The listing builds one solid part. Answer for the finished solid, in the listing's coordinates (mm). Give positions to 0.01 mm unless a question says otherwise; leave off trailing zeros. Order: outer loops, then holes, each group sorted by start corner. A loop starts at its lowest first (then second) coordinate and runs counter-clockwise, first axis right, second up. Notation, with made-up numbers: (20, -8.5) - (35, -8.5) arc R19 cw to (35, -0.5) - close; hole circle Ø6 at (-7.75, -5.75). An arc over 180 degrees is marked (long way). Write each question's results on one line, items separated by ' | '. Start each with the question number.
1. Determine the mould class of faces 1 (the face through (22.1, -9.1, 30)), 2 (the face through (-2.18, 16.61, 9.26)), 3 (the face through (0, 0, 1)) for opening direction Y: released by +Y, released by -Y, zero draft, split by the parting line, or undercut.
2. Section B-B (x = 0) is taken. Give the vertices of the cut face in (y, z), and give its area (3 significant figures).
3. Section C-C (z = 13) is taken. State how many separate pieces and enclosed holes the cut face has, and give its area (3 significant figures).
4. Flat-ended cylindrical pins translate along their axes: pin 1 (2 mm diameter, centred on y = 12.5, z = 23.5, fed in from +X); pin 2 (12 mm diameter, centred on x = 16.5, z = 9, fed in from -Y); pin 3 (5 mm diameter, centred on y = -17, z = 26, fed in from +X). Find the tip coordinate at first contact, or state that the pin passes through.
5. Section A-A (y = 0) is taken. Give the vertices of the cut face in (x, z).
6. Find the intervals of material crossed by L1, parallel to Y at x = 5.5, z = 15; L2, parallel to Y at x = -4, z = 7; L3, parallel to Z at x = 7, y = 7.5, in increasing order.
from build123d import *

# Parameters (mm, degrees)
TORUS_R = 2


with BuildPart() as cono001:
    # Cone001 → Cone001 (revolve)
    with BuildSketch(Plane(origin=(0, 0, 1), x_dir=(1, 0, 0), z_dir=(0, -1, 0))):
        Polygon((0, 0), (14, 0), (24, 30), (0, 30), align=None)
    revolve(axis=Axis((0, 0, 1), (0, 0, 1)))


with BuildPart() as toro:
    # Torus → Torus (revolve)
    with BuildSketch(Plane(origin=(0, -22, 15), x_dir=(0, 0, -1), z_dir=(0, -1, 0))):
        with Locations((10, 0)):
            Circle(TORUS_R)
    revolve(axis=Axis((0, -22, 15), (1, 0, 0)))


with BuildPart() as cut:
    # Cone → Cone (revolve)
    with BuildSketch(Plane.XZ):
        Polygon((0, 0), (15, 0), (25, 30), (0, 30), align=None)
    revolve(axis=Axis((0, 0, 0), (0, 0, 1)))

    # Fusion: union Toro
    add(toro.part)

    # Cut: cut Cono001
    add(cono001.part, mode=Mode.SUBTRACT)


solid = cut.part
Reported:
1) face 1: zero draft | face 2: undercut | face 3: undercut
2) outline: (-25, 30) - (-23.95, 26.84) arc R12 ccw (long way) to (-16.45, 4.36) - (-15, 0) - (15, 0) - (25, 30) - (23.67, 30) - (14, 1) - (-14, 1) - (-23.67, 30) - close; hole (-22.66, 22.97) arc R8 ccw (long way) to (-17.74, 8.23) - close | area: 249 mm²
3) separate pieces: 2 | enclosed holes: 1 | area: 169 mm²
4) pin 1: x = 19.84 | pin 2: y = -15.27 | pin 3: x = 18.97
5) outline: (-25, 30) - (-15, 0) - (15, 0) - (25, 30) - (23.67, 30) - (14, 1) - (-14, 1) - (-23.67, 30) - close
6) L1: -19.23 to -17.84, 17.84 to 19.23 | L2: -16.87 to -15.49, 15.49 to 16.87 | L3: 0 to 1
